Can you work these out from the model? Positions are in its coordinate system, mm. A direction names the side the tool comes from. Coordinates: 2 decimals unless noted, no trailing zeros. Order: outer loops, then holes, each group sorted by start corner. A loop starts at its lowest first (then second) coordinate and runs counter-clockwise, first axis right, second up. Notation, with made-up numbers: (0.5, -32.5) -> (43.5, -32.5) arc R6 ccw to (43.5, -23.5) -> close; hole circle Ø4 at (61, -10). An arc over 180 degrees is marked (long way). Answer as a JSON object with one key per item and string values. Group by question number.
(1) I want a section at B-B, the plane y = 4. List the corners of the cut face in (x, z) for me, plus the area to 3 significant figures.
(2) I want a section at D-D, the plane y = 23.5. List the corners of the cut face in (x, z) for me, plus the area to 3 significant figures.
(3) If we mould it in two halves opening along X, with no side actions, what happens to faces 1 (the cylindrical face through (-15, 3, -57)), 2 (the cylindrical face through (-10.386, 20.325, -38.872)), 3 (the flat face through (-15, 2, 0)), 4 (the flat face through (-15, 5, -80))? For each: pulls with the +X half, pulls with the -X half, needs draft (parallel to the pull), parting line crosses it, or undercut.
(4) I need wall thicknesses on line 1 (Z direction, x = -15, y = 2.6); line 2 (Z direction, x = -9, y = 25); line 3 (X direction, y = 26.5, z = -30). Which ranges of each line are inside material? Lowest first, please.
(5) I want a section at A-A, the plane z = -100. List the corners of the cut face in (x, y) for me.
(6) Which directions (+Z, -Z, +X, -X, +Y, -Y) give clear straight access to the entire face, cutting with the end or side of a thin tool? Please do faces 5 (the cylindrical face through (-15.46, 19.79, -26.53)), 6 (the flat face through (0, 2, -56)).
(7) For pin 1 (2.5 mm diameter, centred on x = -17, z = -78.5, fed in from +Y); pin 2 (3.5 mm diameter, centred on x = -15, z = -55, fed in from -Y); pin 3 (5 mm diameter, centred on x = -5.5, y = 17.5, fed in from -Z); pin 4 (8 mm diameter, centred on y = 29, z = -32.5, fed in from +X), each with a flat end and sliding along its axis, tell me the tip position at first contact or that it passes through.
(8) I want a section at C-C, the plane z = -30. List the corners of the cut face in (x, y) for me, plus the area to 3 significant figures.
Autodesk Inventor part; units mm, degrees
ref_plane "YZ Plane" through (0, 0, 0) normal (1, 0, 0) x (0, 1, 0)
ref_plane "XZ Plane" through (0, 0, 0) normal (0, 1, 0) x (-1, 0, 0)
ref_plane "XY Plane" through (0, 0, 0) normal (0, 0, 1) x (1, 0, 0)
sketch "Sketch1" plane through (0, 0, 0) normal (0, 1, 0) x (-1, 0, 0)
  line L0 (0, 0) -> (30, 0)
  line L1 (30, 0) -> (30, -110)
  line L2 (30, -110) -> (0, -110)
  line L3 (0, -110) -> (0, 0)
  dimension "d0" = 30
  dimension "d1" = 110
extrude "Extrusion1" add sketch "Sketch1" along normal blind 5
sketch "Sketch2" plane through (0, 5, 0) normal (0, 1, 0) x (1, 0, 0)
  circle A0 centre (-10, 30) radius 3.5
  line L0 (0, 0) -> (0, 110)
  line L1 (-30, 0) -> (0, 0)
  circle A1 centre (-10, 30) radius 20
  line L2 (-30, 110) -> (-30, 0)
  circle A2 centre (-15, 10) radius 2
  line L3 (-30, 55) -> (0, 55) construction
  circle A3 centre (-10, 80) radius 3.5
  circle A4 centre (-10, 80) radius 20
  circle A5 centre (-15, 100) radius 2
  circle A6 centre (-15, 55) radius 2
  line L4 (-15, 0) -> (-15, 110) construction
  dimension "d4" = 7
  dimension "d5" = 10
  dimension "d6" = 30
  dimension "d7" = 4
  dimension "d9" = 10
  dimension "d10" = 4
extrude "Extrusion2" cut sketch "Sketch2" against normal blind 5 contours A2 A1 | A1 A2 | A5 A4 | A4 A5 | A6
sketch "Sketch3" plane through (0, 5, 0) normal (0, 1, 0) x (1, 0, 0)
  line L0 (0, 110) -> (0, 0) construction
  line L1 (0, 55) -> (-30, 55) construction
  line L2 (-30, 0) -> (-30, 110) construction
  circle A0 centre (-15, 30) radius 3.5
  circle A1 centre (-15, 80) radius 4.1
  line L3 (-30, 0) -> (0, 0)
  line L4 (0, 110) -> (-30, 110)
  circle A2 centre (-15, 30) radius 10
  circle A3 centre (-15, 80) radius 10
  line L5 (-30, 110) -> (-30, 0)
  line L6 (-15, 0) -> (-15, 110) construction
  dimension "d13" = 7
  dimension "d14" = 8.2
  dimension "d16" = 30
  dimension "d17" = 30
  dimension "d22" = 20
extrude "Extrusion3" add sketch "Sketch3" along normal blind 30
chamfer "Chamfer1" distance 3 angle 45 1 edges at (-25, 5, -30)
chamfer "Chamfer2" distance 3 angle 45 1 edges at (-25, 5, -80)
chamfer "Chamfer3" distance 3 angle 45 4 edges at (-30, 2.5, 0) (0, 2.5, 0) (0, 2.5, -110) (-30, 2.5, -110)
chamfer "Chamfer4" distance 2 angle 45 2 edges at (-25, 35, -80) (-25, 35, -30)
Computed values:
{
 "1": {"outline": "(-30, -107) -> (-27, -110) -> (-3, -110) -> (0, -107) -> (0, -3) -> (-3, 0) -> (-27, 0) -> (-30, -3) -> close; hole circle Ø4 at (-15, -100); hole circle Ø4 at (-15, -55); hole circle Ø4 at (-15, -10)", "area": "3,240 mm2"},
 "2": {"outline": "circle Ø20 at (-15, -80); circle Ø20 at (-15, -30); hole circle Ø8.2 at (-15, -80); hole circle Ø7 at (-15, -30)", "area": "537 mm2"},
 "3": {"face 1": "undercut", "face 2": "parting line crosses it", "face 3": "needs draft", "face 4": "undercut"},
 "4": {"line 1": "z = -110 to -102, -98 to -57, -53 to -12, -8 to 0", "line 2": "z = -88 to -72, -38 to -22", "line 3": "x = -25 to -18.5, -11.5 to -5"},
 "5": {"outline": "(-30, 0) -> (-17, 0) -> (-17, 5) -> (-30, 5) -> close; (-13, 0) -> (0, 0) -> (0, 5) -> (-13, 5) -> close"},
 "6": {"face 5": "+Y", "face 6": "+Z, -Z, +X, +Y, -Y"},
 "7": {"pin 1": "stops at y = 5", "pin 2": "passes through", "pin 3": "stops at z = -87.14", "pin 4": "stops at x = -5"},
 "8": {"outline": "(-30, 0) -> (0, 0) -> (0, 5) -> (-2, 5) -> (-5, 8) -> (-5, 33) -> (-7, 35) -> (-11.5, 35) -> (-11.5, 5) -> (-18.5, 5) -> (-18.5, 35) -> (-23, 35) -> (-25, 33) -> (-25, 8) -> (-28, 5) -> (-30, 5) -> close", "area": "545 mm2"}
}
